CAD build for the part. Positions are in the model's coordinates, mm. Face numbers are marked on the shaded views. A direction names the side the tool comes from. Round coordinates to 2 decimals unless told otherwise and drop trailing zeros. Loops run counter-clockwise (first coordinate to the right, second up) from the corner with the lowest first, then second, coordinate; pieces in that order, holes last.
```python
from build123d import *

# Parameters (mm, degrees)
F1_DEPTH = 7.7


with BuildPart() as f1:
    # F0 (on Top) → F1 (new body)
    with BuildSketch(Plane.XY):
        with BuildLine():
            add(Edge.make_bspline(
                [(22.0934028303, -3.5129354261), (22.2431585024, -3.6009011816), (22.3875659726, -3.6886724571)],
                knots=[0.9635630597, 0.9635630597, 0.9635630597, 1, 1, 1], degree=2))
            ThreePointArc((22.0934028303, -3.5129354261), (21.1126986682, -7.6642760258), (19.0031102486, -11.3717072292))
            add(Edge.make_bspline(
                [(19.2055998268, -11.5662766238), (19.1082850147, -11.4689618118), (19.0031102486, -11.3717072292)],
                knots=[0, 0, 0, 0.0430145471, 0.0430145471, 0.0430145471], degree=2))
            add(Edge.make_bspline(
                [(21.4679696184, -17.4907557905), (21.4679696184, -13.8286464155), (19.2055998268, -11.5662766238)],
                knots=[0, 0, 0, 1, 1, 1], degree=2))
            add(Edge.make_bspline(
                [(10.4328133684, -26.8494797488), (21.4679696184, -25.3358078738), (21.4679696184, -17.4907557905)],
                knots=[0, 0, 0, 1, 1, 1], degree=2))
            Line((10.4328133684, -26.8494797488), (10.4328133684, -16.8120794212))
            ThreePointArc((10.4328133684, -16.8120794212), (7.1531909726, -17.1750005821), (3.8735685768, -16.8120794212))
            Line((3.8735685768, -16.8120794212), (3.8735685768, -27.3703130821))
            add(Edge.make_bspline(
                [(-6.1687491316, -26.1740240196), (-0.6511710066, -27.3703130821), (3.8735685768, -27.3703130821)],
                knots=[0, 0, 0, 1, 1, 1], degree=2))
            add(Edge.make_bspline(
                [(-15.9180980899, -23.0897141238), (-11.6863272566, -24.9777349571), (-6.1687491316, -26.1740240196)],
                knots=[0, 0, 0, 1, 1, 1], degree=2))
            Line((-15.9180980899, -23.0897141238), (-15.9180980899, -31.0324224571))
            add(Edge.make_bspline(
                [(-7.1615876732, -33.4982427696), (-12.5001293399, -32.6111984988), (-15.9180980899, -31.0324224571)],
                knots=[0, 0, 0, 1, 1, 1], degree=2))
            add(Edge.make_bspline(
                [(3.8735685768, -34.3852870405), (-1.8230460066, -34.3852870405), (-7.1615876732, -33.4982427696)],
                knots=[0, 0, 0, 1, 1, 1], degree=2))
            Line((3.8735685768, -34.3852870405), (3.8735685768, -45.7296880821))
            Line((3.8735685768, -45.7296880821), (10.4328133684, -45.7296880821))
            Line((10.4328133684, -45.7296880821), (10.4328133684, -33.9295578738))
            add(Edge.make_bspline(
                [(24.9347664934, -28.257357353), (19.7427092018, -32.7576828738), (10.4328133684, -33.9295578738)],
                knots=[0, 0, 0, 1, 1, 1], degree=2))
            add(Edge.make_bspline(
                [(30.1268237851, -16.8397141238), (30.1268237851, -23.7570318321), (24.9347664934, -28.257357353)],
                knots=[0, 0, 0, 1, 1, 1], degree=2))
            add(Edge.make_bspline(
                [(28.2388029518, -9.2306646446), (30.1268237851, -12.3638026655), (30.1268237851, -16.8397141238)],
                knots=[0, 0, 0, 1, 1, 1], degree=2))
            add(Edge.make_bspline(
                [(22.3875659726, -3.6886724571), (26.3507821184, -6.0975266238), (28.2388029518, -9.2306646446)],
                knots=[0, 0, 0, 1, 1, 1], degree=2))
        make_face()
        with BuildLine():
            ThreePointArc((3.8735685768, 12.4620782569), (7.1531909726, 12.8249994179), (10.4328133684, 12.4620782569))
            Line((10.4328133684, 12.4620782569), (10.4328133684, 23.3458327512))
            add(Edge.make_bspline(
                [(25.8462248268, 19.7813796262), (18.2615894101, 22.7924473345), (10.4328133684, 23.3458327512)],
                knots=[0, 0, 0, 1, 1, 1], degree=2))
            Line((25.8462248268, 19.7813796262), (28.4992196184, 26.4545567095))
            add(Edge.make_bspline(
                [(10.4328133684, 30.2143223345), (19.7915373268, 29.9539056679), (28.4992196184, 26.4545567095)],
                knots=[0, 0, 0, 1, 1, 1], degree=2))
            Line((10.4328133684, 30.2143223345), (10.4328133684, 39.3614577512))
            Line((10.4328133684, 39.3614577512), (3.8735685768, 39.3614577512))
            Line((3.8735685768, 39.3614577512), (3.8735685768, 30.1166660845))
            add(Edge.make_bspline(
                [(-9.7820303816, 24.916470772), (-4.6225251732, 29.1889317095), (3.8735685768, 30.1166660845)],
                knots=[0, 0, 0, 1, 1, 1], degree=2))
            add(Edge.make_bspline(
                [(-14.9415355899, 13.9871087929), (-14.9415355899, 20.6440098345), (-9.7820303816, 24.916470772)],
                knots=[0, 0, 0, 1, 1, 1], degree=2))
            add(Edge.make_bspline(
                [(-10.7504548607, 2.6915358762), (-14.9415355899, 7.0697910845), (-14.9415355899, 13.9871087929)],
                knots=[0, 0, 0, 1, 1, 1], degree=2))
            add(Edge.make_bspline(
                [(-7.6647341063, 0.1550415541), (-9.489916275, 1.3747013925), (-10.7504548607, 2.6915358762)],
                knots=[0.6992330458, 0.6992330458, 0.6992330458, 1, 1, 1], degree=2))
            ThreePointArc((-7.6647341063, 0.1550415541), (-6.3961953475, 4.2603805526), (-4.0158241247, 7.8376465082))
            add(Edge.make_bspline(
                [(-4.0610017357, 7.8835931679), (-4.038574566, 7.8606073142), (-4.0158241247, 7.8376465082)],
                knots=[0, 0, 0, 0.0098072976, 0.0098072976, 0.0098072976], degree=2))
            add(Edge.make_bspline(
                [(-6.3477855899, 14.0847650429), (-6.3477855899, 10.2273431679), (-4.0610017357, 7.8835931679)],
                knots=[0, 0, 0, 1, 1, 1], degree=2))
            add(Edge.make_bspline(
                [(-3.7517569441, 19.9604160845), (-6.3477855899, 17.6003900429), (-6.3477855899, 14.0847650429)],
                knots=[0, 0, 0, 1, 1, 1], degree=2))
            add(Edge.make_bspline(
                [(3.8735685768, 23.1342442095), (-1.1557282982, 22.3204421262), (-3.7517569441, 19.9604160845)],
                knots=[0, 0, 0, 1, 1, 1], degree=2))
            Line((3.8735685768, 23.1342442095), (3.8735685768, 12.4620782569))
        make_face()
        with BuildLine():
            ThreePointArc((3.8735685768, -16.8120794212), (7.1531909726, -17.1750005821), (10.4328133684, -16.8120794212))
            Line((10.4328133684, -16.8120794212), (10.4328133684, -12.622324495))
            ThreePointArc((10.4328133684, -12.622324495), (7.1531909726, -13.1250005821), (3.8735685768, -12.622324495))
            Line((3.8735685768, -12.622324495), (3.8735685768, -16.8120794212))
        make_face()
        with BuildLine():
            Line((10.4328133684, 8.2723233307), (10.4328133684, 12.4620782569))
            ThreePointArc((10.4328133684, 12.4620782569), (7.1531909726, 12.8249994179), (3.8735685768, 12.4620782569))
            Line((3.8735685768, 12.4620782569), (3.8735685768, 8.2723233307))
            ThreePointArc((3.8735685768, 8.2723233307), (7.1531909726, 8.7749994179), (10.4328133684, 8.2723233307))
        make_face()
        with BuildLine():
            ThreePointArc((19.0031102486, -11.3717072292), (21.1126986682, -7.6642760258), (22.0934028303, -3.5129354261))
            add(Edge.make_bspline(
                [(18.0838779902, -1.5249380293), (20.4218137777, -2.5310521228), (22.0934028303, -3.5129354261)],
                knots=[0.5568499804, 0.5568499804, 0.5568499804, 0.9635630597, 0.9635630597, 0.9635630597], degree=2))
            ThreePointArc((18.0838779902, -1.5249380293), (18.0983616621, -1.849825893), (18.1031909726, -2.1750005821))
            ThreePointArc((18.1031909726, -2.1750005821), (17.4541754224, -5.8887883204), (15.584064148, -9.1623375213))
            add(Edge.make_bspline(
                [(19.0031102486, -11.3717072292), (17.8042308259, -10.2631093973), (15.584064148, -9.1623375213)],
                knots=[0.0430145471, 0.0430145471, 0.0430145471, 0.5333342058, 0.5333342058, 0.5333342058], degree=2))
        make_face()
        with BuildLine():
            add(Edge.make_bspline(
                [(-4.0158241247, 7.8376465082), (-2.8074328759, 6.6180817259), (-0.6870243927, 5.4691817173)],
                knots=[0.0098072976, 0.0098072976, 0.0098072976, 0.5307225792, 0.5307225792, 0.5307225792], degree=2))
            ThreePointArc((-4.0158241247, 7.8376465082), (-6.3961953475, 4.2603805526), (-7.6647341063, 0.1550415541))
            add(Edge.make_bspline(
                [(-3.7957490763, -2.0226463711), (-5.9728358213, -0.9755526541), (-7.6647341063, 0.1550415541)],
                knots=[0.4204295912, 0.4204295912, 0.4204295912, 0.6992330458, 0.6992330458, 0.6992330458], degree=2))
            ThreePointArc((-3.7957490763, -2.0226463711), (-2.960659052, 2.0217288206), (-0.6870243927, 5.4691817173))
        make_face()
        with BuildLine():
            add(Edge.make_bspline(
                [(-3.7957490763, -2.0226463711), (-5.9728358213, -0.9755526541), (-7.6647341063, 0.1550415541)],
                knots=[0.4204295912, 0.4204295912, 0.4204295912, 0.6992330458, 0.6992330458, 0.6992330458], degree=2))
            ThreePointArc((-7.6647341063, 0.1550415541), (-5.2504820599, -10.6099810387), (3.8735685768, -16.8120794212))
            Line((3.8735685768, -16.8120794212), (3.8735685768, -12.622324495))
            ThreePointArc((3.8735685768, -12.622324495), (-1.7181838585, -8.5938173427), (-3.7957490763, -2.0226463711))
        make_face()
        with BuildLine():
            ThreePointArc((10.4328133684, -16.8120794212), (15.1921691537, -14.8389190043), (19.0031102486, -11.3717072292))
            add(Edge.make_bspline(
                [(19.0031102486, -11.3717072292), (17.8042308259, -10.2631093973), (15.584064148, -9.1623375213)],
                knots=[0.0430145471, 0.0430145471, 0.0430145471, 0.5333342058, 0.5333342058, 0.5333342058], degree=2))
            ThreePointArc((15.584064148, -9.1623375213), (13.2586642627, -11.2648683427), (10.4328133684, -12.622324495))
            Line((10.4328133684, -12.622324495), (10.4328133684, -16.8120794212))
        make_face()
        with BuildLine():
            ThreePointArc((22.0934028303, -3.5129354261), (22.1382364825, -2.8446356075), (22.1531909726, -2.1750005821))
            ThreePointArc((22.1531909726, -2.1750005821), (18.8620409575, 7.2006504369), (10.4328133684, 12.4620782569))
            Line((10.4328133684, 12.4620782569), (10.4328133684, 8.2723233307))
            ThreePointArc((10.4328133684, 8.2723233307), (15.783359334, 4.5646354655), (18.0838779902, -1.5249380293))
            add(Edge.make_bspline(
                [(18.0838779902, -1.5249380293), (20.4218137777, -2.5310521228), (22.0934028303, -3.5129354261)],
                knots=[0.5568499804, 0.5568499804, 0.5568499804, 0.9635630597, 0.9635630597, 0.9635630597], degree=2))
        make_face()
        with BuildLine():
            Line((3.8735685768, 8.2723233307), (3.8735685768, 12.4620782569))
            ThreePointArc((3.8735685768, 12.4620782569), (-0.4321319343, 10.7657442341), (-4.0158241247, 7.8376465082))
            add(Edge.make_bspline(
                [(-4.0158241247, 7.8376465082), (-2.8074328759, 6.6180817259), (-0.6870243927, 5.4691817173)],
                knots=[0.0098072976, 0.0098072976, 0.0098072976, 0.5307225792, 0.5307225792, 0.5307225792], degree=2))
            ThreePointArc((-0.6870243927, 5.4691817173), (1.4193354909, 7.153740025), (3.8735685768, 8.2723233307))
        make_face()
    extrude(amount=F1_DEPTH)


solid = f1.part
```
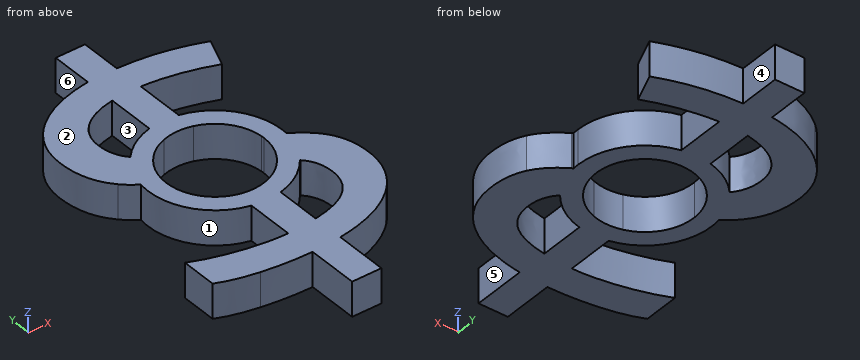
Item 1: Cut at B-B, the plane z = 2.25. State how many separate pieces and enclosed holes the cut face has, plus the area to 3 significant figures.
Answers follow:
separate pieces: 1
enclosed holes: 3
area: 1,490 mm2
Item 2: 3-axis set-ups, long thin cutter, end or side, ignore diameter. For the marked faces 4, 5 and 6: which of +Z, -Z, +X, -X, +Y, -Y reach the whole face in a straight line?
Answers follow:
face 4: +Z, -Z, +X, +Y
face 5: +Z, -Z, +X, -Y
face 6: +Z, -Z, -X, +Y
Item 3: Flat gauge pins, fed straight in: P1, Ø4, axis at y = -20.5, z = 5.5, coming from the -X side; P2, Ø2.5, axis at y = -39, z = 5.5, coming from the +X side; P3, Ø2, axis at x = 14.5, z = 3.5, coming from the -Y side. Where does each tip first touch, or does it go through?
Answers follow:
P1: stops at x = 3.87
P2: stops at x = 10.43
P3: stops at y = -33.43
Item 4: Probe line 1 (Y direction, x = 13.5, z = 1.25); line 2 (Y direction, x = 13, z = 4); line 3 (X direction, y = -19, z = 3.75). List the from-to ranges inside material, lowest first.
Answers follow:
line 1: y = -33.43 to -26.25, -15.77 to -11.1, 6.75 to 11.42, 23.03 to 30.04
line 2: y = -33.53 to -26.38, -15.99 to -11.43, 7.08 to 11.64, 23.1 to 30.08
line 3: x = 3.87 to 10.43, 21.36 to 29.99
Item 5: Two-plate mould, pull along X, no slides. Class the marked faces 1, 2 and 3: released by +X, released by -X, zero draft, split by the parting line, or undercut.
Answers follow:
face 1: released by -X
face 2: zero draft
face 3: undercut
Item 6: Cut at A-A, the plane x = 8. Give the cut face in (y, z).
Answers follow:
outline: (-45.73, 0) - (-13.09, 0) - (-13.09, 7.7) - (-45.73, 7.7) - close; (8.74, 0) - (39.36, 0) - (39.36, 7.7) - (8.74, 7.7) - close
